Part model, mm, in its own coordinate system. A direction names the side the tool comes from. Round coordinates to 2 decimals unless told otherwise and drop trailing zeros. Write each loop counter-clockwise with the first axis right and the second up, starting at its lowest first coordinate (ties: lowest second). Pieces come first, ordered by that corner, then holes. Notation, with made-up numbers: M 69.25,-34.5 L 124.25,-34.5 A26 cw 124.25,-17.5 Z; hole C 34,18.5 d1. An arc over 180 degrees is marked long. Use a Markdown table: item, result. Add a question column.
1) Two-plate mould, pull along X, no slides. Class faces 1 (the face through (9.75, 0, 2)), 2 (the face through (0.75, -5, 4)), 3 (the face through (0.1, -9.75, 0.7)): released by +X, released by -X, zero draft, split by the parting line, or undercut.
2) Drop flat-ended pins along their axis: P1, Ø0.8, axis at x = 0, y = -10.5, coming from the +Z side; P2, Ø5, axis at x = -3.5, y = 2, coming from the -Z side; P3, Ø1.3, axis at x = 4.5, z = 1, coming from the -Y side; P4, Ø2, axis at x = 4.5, y = -6, coming from the +Z side. Give the stop position or say it passes through.
3) Slice it at A-A on y = -1.75. Write the cut outline in (x, z).
4) Wall check: probe 1 along Y at (x, z) = (5.25, 3.7); probe 2 along X at (y, z) = (-2, 0.25). Give the ranges that are in metal, low to high.
5) Slice it at B-B on z = 1.95. Write the cut outline in (x, y), plus the area to 4 significant figures.
6) Which spindle directions (+Z, -Z, +X, -X, +Y, -Y) get a long thin tool onto all of the face, cutting with end or side? Do faces 4 (the face through (0, 9.75, 2)), 5 (the face through (5, -11, 3)), 6 (the face through (0, -11, 0.988)), 7 (the face through (-5, -11, 3)), 8 (the face through (5, 0.75, 4)). Say none if no direction does.
7) Slice it at D-D on x = 2.75. Give the number of separate pieces and of enclosed holes in the cut face, plus the area to 3 significant figures.
Autodesk Fusion 360 part; units mm, degrees
sketch "Sketch1" plane through (0, 0, 0) normal (0, 0, 1) x (1, 0, 0)
  line L0 (8.75, -8.75) -> (-8.75, -8.75)
  line L1 (-8.75, -8.75) -> (-8.75, 8.75)
  line L2 (-8.75, 8.75) -> (8.75, 8.75)
  line L3 (8.75, 8.75) -> (8.75, -8.75)
  line L4 (8.75, -8.75) -> (-8.75, 8.75) construction
  line L5 (-8.75, -8.75) -> (8.75, 8.75) construction
  line L6 (9.75, -9.75) -> (-9.75, -9.75)
  line L7 (-9.75, -9.75) -> (-9.75, 9.75)
  line L8 (-9.75, 9.75) -> (9.75, 9.75)
  line L9 (9.75, 9.75) -> (9.75, -9.75)
  line L10 (9.75, -9.75) -> (-9.75, 9.75) construction
  line L11 (-9.75, -9.75) -> (9.75, 9.75) construction
  dimension "d1" = 17.5
  dimension "d2" = 17.5
  dimension "d3" = 19.5
  dimension "d4" = 19.5
extrude "Extrude1" add sketch "Sketch1" along normal blind 3.5
sketch "Sketch2" plane through (0, 0, 3.5) normal (0, 0, 1) x (-1, 0, 0)
  line L0 (8.75, -8.75) -> (-8.75, -8.75)
  line L1 (-8.75, -8.75) -> (-8.75, 8.75)
  line L2 (-8.75, 8.75) -> (8.75, 8.75)
  line L3 (8.75, 8.75) -> (8.75, -8.75)
  line L4 (-9.75, -9.75) -> (9.75, -9.75)
  line L5 (9.75, -9.75) -> (9.75, 9.75)
  line L6 (9.75, 9.75) -> (-9.75, 9.75)
  line L7 (-9.75, 9.75) -> (-9.75, -9.75)
  line L8 (0.75, -9.75) -> (-0.75, -9.75)
  line L9 (-0.75, -9.75) -> (-0.75, 9.75)
  line L10 (-0.75, 9.75) -> (0.75, 9.75)
  line L11 (0.75, 9.75) -> (0.75, -9.75)
  line L12 (0.75, -9.75) -> (-0.75, 9.75) construction
  line L13 (-0.75, -9.75) -> (0.75, 9.75) construction
  line L14 (9.75, -0.75) -> (-9.75, -0.75)
  line L15 (-9.75, -0.75) -> (-9.75, 0.75)
  line L16 (-9.75, 0.75) -> (9.75, 0.75)
  line L17 (9.75, 0.75) -> (9.75, -0.75)
  line L18 (9.75, -0.75) -> (-9.75, 0.75) construction
  line L19 (-9.75, -0.75) -> (9.75, 0.75) construction
  dimension "d7" = 1.5
  dimension "d8" = 1.5
extrude "Extrude2" add sketch "Sketch2" along normal blind 1 contours L0 L3 L4 L5 L11 L14 | L0 L4 L8 L9 L11 | L0 L9 L11 L14 | L3 L11 L14 L16 | L3 L5 L14 L16 L17 | L0 L1 L4 L7 L9 L14 | L9 L11 L14 L16 | L2 L3 L5 L6 L11 L16 | L1 L9 L14 L16 | L2 L9 L11 L16 | L1 L7 L14 L15 L16 | L2 L6 L9 L10 L11 | L1 L2 L6 L7 L9 L16
ref_plane "WorkPlane1" through (0, 0, 2.25) normal (1, 0, 0) x (0, 1, 0)
sketch "Sketch3" plane through (0, 0, 2.25) normal (1, 0, 0) x (0, 1, 0)
  line L0 (-9.7484, 2.2378) -> (-12.4984, 2.2378)
  line L1 (-12.4984, 2.2378) -> (-12.4984, -0.5122)
  line L2 (-12.4984, -0.5122) -> (-9.7484, -0.5122)
  line L3 (-9.7484, -0.5122) -> (-9.7484, 2.2378)
  circle A0 centre (-12.4831, 0.4878) radius 1.75
  circle A1 centre (-12.4831, 0.4878) radius 1.2499
  line L4 (-9.7484, -0.5122) -> (-12.4754, -0.5122)
  line L5 (-12.4754, -0.5122) -> (-12.4754, -1.2622)
  line L6 (-12.4754, -1.2622) -> (-9.7484, -1.2622)
  line L7 (-9.7484, -1.2622) -> (-9.7484, -0.5122)
  dimension "d12" = 2.75
  dimension "d13" = 2.75
  dimension "d14" = 3.5
  dimension "d15" = 2.4999
extrude "Extrude3" add sketch "Sketch3" along normal blind 5 contours L1 L2 A0 A1 L4 | L1 A0 A1 L5 | L0 L2 L3 A0 L4 | L2 A0 L4 L6 L7 | L2 A0 A1 L4 L5
extrude "Extrude4" add sketch "Sketch3" against normal blind 5 contours L1 L2 A0 A1 L4 | L1 A0 A1 L5 | L0 L2 L3 A0 L4 | L2 A0 L4 L6 L7 | L2 A0 A1 L4 L5
Entries:
| question | item | result |
|---|---|---|
| 1 | face 1 | released by +X |
| 1 | face 2 | undercut |
| 1 | face 3 | zero draft |
| 2 | P1 | stops at z = 4.49 |
| 2 | P2 | stops at z = 3.5 |
| 2 | P3 | stops at y = -13.85 |
| 2 | P4 | passes through |
| 3 | outline | M -9.75,0 L -8.75,0 L -8.75,4.5 L -9.75,4.5 Z; M -0.75,3.5 L 0.75,3.5 L 0.75,4.5 L -0.75,4.5 Z; M 8.75,0 L 9.75,0 L 9.75,4.5 L 8.75,4.5 Z |
| 4 | probe 1 | y = -9.75 to -8.75, -0.75 to 0.75, 8.75 to 9.75 |
| 4 | probe 2 | x = -9.75 to -8.75, 8.75 to 9.75 |
| 5 | outline | M -9.75,-9.75 L -5,-9.75 L -5,-11.51 L 5,-11.51 L 5,-9.75 L 9.75,-9.75 L 9.75,9.75 L -9.75,9.75 Z; M -5,-14.05 L 5,-14.05 L 5,-13.45 L -5,-13.45 Z; hole M -8.75,-8.75 L 8.75,-8.75 L 8.75,8.75 L -8.75,8.75 Z |
| 5 | area | 97.55 mm^2 |
| 6 | face 4 | +Z, -Z, +X, -X, +Y |
| 6 | face 5 | +Z, -Z, +X, -Y |
| 6 | face 6 | -Z, +X, -X, -Y |
| 6 | face 7 | +Z, -Z, -X, -Y |
| 6 | face 8 | +Z, -Z |
| 7 | separate pieces | 3 |
| 7 | enclosed holes | 1 |
| 7 | area | 20.0 mm^2 |
